Source: CAD feature listing. Evaluate the final solid. Frame: model axes, mm. Face numbers are marked on the shaded views. Give positions to 0.01 mm unless a question says otherwise; leave off trailing zeros. Loops run counter-clockwise (first coordinate to the right, second up) from the corner with the lowest first, then second, coordinate; pieces in that order, holes last. Notation, with made-up numbers: (-28, -18.5) -> (30, -18.5) arc R32 cw to (30, 19.5) -> close; hole circle Ø1 at (70.5, 52). An arc over 180 degrees is marked (long way). Put each result on its own line as item: value.
```python
from build123d import *

# Parameters (mm, degrees)
SKETCH1_W             = 35
SKETCH1_H             = 47.5
SKETCH1_R             = 2.5
BOSS_EXTRUDE1_DEPTH   = 4.7625
F_4_CLEARANCE_HOLE1_D = 3.2639
FILLET1_R             = 5
F_4_CLEARANCE_HOLE2_D = 3.2639


with BuildPart() as part:
    # Sketch1 → Boss-Extrude1 (new body)
    with BuildSketch(Plane.XY):
        Rectangle(SKETCH1_W, SKETCH1_H)
        with Locations(Location((10, 8.75, 0), (0, 0, 180))):
            Circle(SKETCH1_R, mode=Mode.SUBTRACT)
    extrude(amount=BOSS_EXTRUDE1_DEPTH)

    # #4 Clearance Hole1 (through all)
    with Locations(Plane.XY.offset(4.7625)):
        with Locations((10, 18.96), (10, -1.46), (-12.17, 8.75)):
            Hole(F_4_CLEARANCE_HOLE1_D / 2)

    # Fillet1
    fillet1_edges = [part.edges().sort_by_distance(p)[0] for p in [
        (-17.5, 23.75, 2.38125),
        (17.5, 23.75, 2.38125),
    ]]
    fillet(fillet1_edges, radius=FILLET1_R)

    # #4 Clearance Hole2 (through all)
    with Locations(Plane.XY.offset(4.7625)):
        with Locations((-12.5, -18.75), (12.5, -18.75), (-5, -18.75), (5, -18.75)):
            Hole(F_4_CLEARANCE_HOLE2_D / 2)


solid = part.part
```
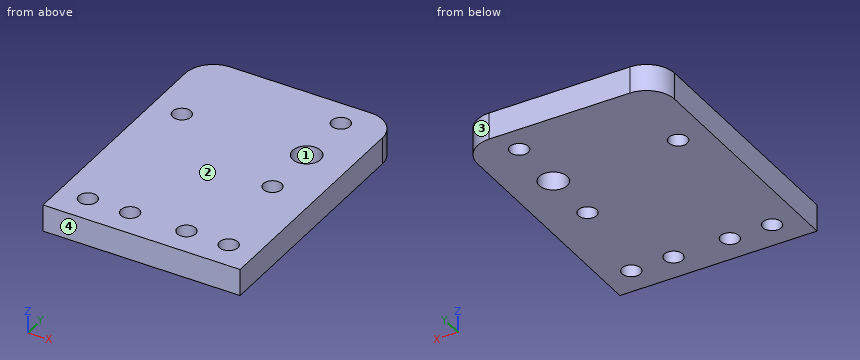
(1) Section A-A on x = -5. Return loops of the section in (y, z).
Calculated:
outline: (-23.75, 0) -> (-20.38, 0) -> (-20.38, 4.76) -> (-23.75, 4.76) -> close; (-17.12, 0) -> (23.75, 0) -> (23.75, 4.76) -> (-17.12, 4.76) -> close
(2) Section B-B on z = 3.9. Give the number of separate pieces and of enclosed holes in the cut face, then the cut area to 3 significant figures.
Calculated:
separate pieces: 1
enclosed holes: 8
area: 1,570 mm²
(3) Line query: probe 1 along X at (y, z) = (8, 0.85); probe 2 along Y at (x, z) = (10, 1.7); probe 3 along Y at (x, z) = (-5, 2.35). Output: solid intervals per line, ascending. Write a range as from..to.
Calculated:
probe 1: x = -17.5..-13.62, -10.72..7.62, 12.38..17.5
probe 2: y = -23.75..-3.09, 0.17..6.25, 11.25..17.33, 20.59..23.75
probe 3: y = -23.75..-20.38, -17.12..23.75
(4) Draft query along Y for the marked faces 1, 2, 3 and 4. Return one class per face: released by +Y, released by -Y, zero draft, split by the parting line, or undercut.
Calculated:
face 1: undercut
face 2: zero draft
face 3: released by +Y
face 4: released by -Y
(5) First-contact query: P1, Ø4, axis at x = 12.5, y = -18.75, coming from the -Z side. Flat tip, straight axial feed; report the tip coordinate or a pass-through.
Calculated:
P1: stops at z = 0
